Check sheet for the modelled part. Datum: model origin and axes. Units: mm. Round coordinates to 2 decimals unless told otherwise and drop trailing zeros. Answer in a Markdown table with one row per item. Add a question column.
(1) Gauge pin test, flat ends, axial feed: pin 1 (3.5 mm diameter, centred on x = 67.66, z = 82.18, fed in from -Y); pin 2 (3.5 mm diameter, centred on x = 83.14, z = -39.84, fed in from -Y); pin 3 (1.5 mm diameter, centred on x = 147.5, y = 2, fed in from +Z); pin 4 (0.9 mm diameter, centred on x = -133, y = 2, fed in from -Z). Record the tip position at first contact, or that the pin passes through.
(2) Cross-section at A-A on y = 1.85. Count the separate pieces of the cut face and the enclosed holes in it, then the cut area to 3 significant figures.
(3) Thickness scan on line 1 along Z through (x, y) = (70, 1.55); line 2 along Z through (x, y) = (-50, 1.8); line 3 along X through (y, z) = (0.6, 118). Record the ranges inside material, lowest first.
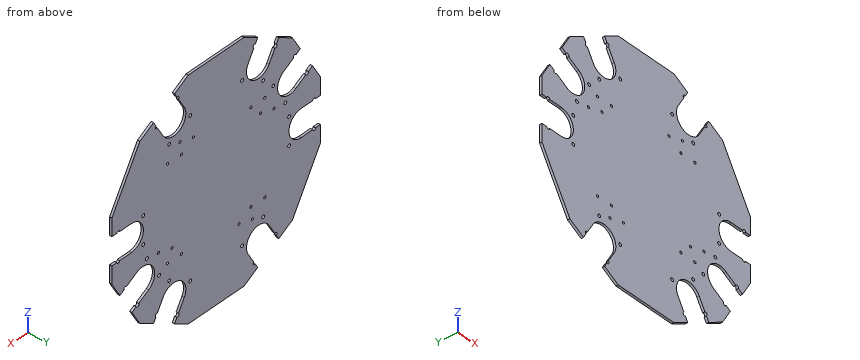
from build123d import *

# Parameters (mm, degrees)
BOSS_EXTRUDE1_DEPTH     = 3
SKETCH2_R               = 2.05
HEXCUT1_DEPTH           = 3
SKETCH5_R               = 1.55
RAILMOUNTHOLES_DEPTH    = 3
LPATTERN1_COUNT         = 2
LPATTERN1_PITCH         = 120
LPATTERN1_COUNT_DIR2    = 2
LPATTERN1_PITCH_DIR2    = 120
SKETCH6_R               = 2.05
QUADCUT1_DEPTH          = 3
CUT_EXTRUDE3_DEPTH      = 3
CUT_EXTRUDE4_DEPTH      = 3
SKETCH9_R               = 1.55
CUT_EXTRUDE5_DEPTH      = 3
MIRROR6_COPY_1_SKETCH_R = 1.55
MIRROR6_COPY_1_DEPTH    = 3
MIRROR6_COPY_2_SKETCH_R = 1.55
MIRROR6_COPY_2_DEPTH    = 3


with BuildPart() as part:
    # Sketch1 → Boss-Extrude1 (new body)
    with BuildSketch(Plane(origin=(0, 0, 0), x_dir=(1, 0, 0), z_dir=(0, 1, 0))):
        Polygon((150, -40.192378865), (150, 40.192378865), (109.807621135, 109.807621135), (40.192378865, 150), (-40.192378865, 150), (-109.807621135, 109.807621135), (-150, 40.192378865), (-150, -40.192378865), (-109.807621135, -109.807621135), (-40.192378865, -150), (40.192378865, -150), (109.807621135, -109.807621135), align=None)
    extrude(amount=BOSS_EXTRUDE1_DEPTH)

    # Sketch2 → HexCut1 (cut)
    with BuildSketch(Plane(origin=(0, 3, 0), x_dir=(1, 0, 0), z_dir=(0, 1, 0))):
        with Locations(Location((55.344555434, 130.859581934, 0), (0, 0, 270))):
            Circle(SKETCH2_R)
        with Locations(Location((37.344555434, 99.682667397, 0), (0, 0, 270))):
            Circle(SKETCH2_R)
        with Locations(Location((37.344555434, -99.682667397, 0), (0, 0, 270))):
            Circle(SKETCH2_R)
        with Locations(Location((55.344555434, -130.859581934, 0), (0, 0, 270))):
            Circle(SKETCH2_R)
        with Locations(Location((105, 17.5, 0), (0, 0, 270))):
            Circle(SKETCH2_R)
        with Locations(Location((141, 17.5, 0), (0, 0, 270))):
            Circle(SKETCH2_R)
        with Locations(Location((105, -17.5, 0), (0, 0, 270))):
            Circle(SKETCH2_R)
        with Locations(Location((141, -17.5, 0), (0, 0, 270))):
            Circle(SKETCH2_R)
        with Locations(Location((85.655444566, -113.359581934, 0), (0, 0, 270))):
            Circle(SKETCH2_R)
        with Locations(Location((67.655444566, -82.182667397, 0), (0, 0, 270))):
            Circle(SKETCH2_R)
        with Locations(Location((85.655444566, 113.359581934, 0), (0, 0, 270))):
            Circle(SKETCH2_R)
        with Locations(Location((67.655444566, 82.182667397, 0), (0, 0, 270))):
            Circle(SKETCH2_R)
    hexcut1 = extrude(amount=-HEXCUT1_DEPTH, mode=Mode.SUBTRACT)

    # HexCut2: HexCut1 across plane
    add(hexcut1.mirror(Plane(origin=(0, 0, 0), x_dir=(0, 0, 1), z_dir=(1, 0, 0))), mode=Mode.SUBTRACT)

    # Sketch5 → RailMountHoles (cut)
    with BuildSketch(Plane(origin=(0, 3, 0), x_dir=(1, 0, 0), z_dir=(0, 1, 0))):
        with Locations(Location((50, 60, 0), (0, 0, 270))):
            Circle(SKETCH5_R)
        with Locations(Location((70, 60, 0), (0, 0, 270))):
            Circle(SKETCH5_R)
    railmountholes = extrude(amount=-RAILMOUNTHOLES_DEPTH, mode=Mode.SUBTRACT)

    # LPattern1: RailMountHoles 2 × 2
    with Locations(*[(-j * LPATTERN1_PITCH_DIR2, 0, i * LPATTERN1_PITCH) for i in range(LPATTERN1_COUNT) for j in range(LPATTERN1_COUNT_DIR2) if (i, j) != (0, 0)]):
        add(railmountholes, mode=Mode.SUBTRACT)

    # Sketch6 → QuadCut1 (cut)
    with BuildSketch(Plane(origin=(0, 3, 0), x_dir=(1, 0, 0), z_dir=(0, 1, 0))):
        with Locations(Location((99.682667397, 37.344555434, 0), (0, 0, 270))):
            Circle(SKETCH6_R)
        with Locations(Location((130.859581934, 55.344555434, 0), (0, 0, 270))):
            Circle(SKETCH6_R)
        with Locations(Location((113.359581934, 85.655444566, 0), (0, 0, 270))):
            Circle(SKETCH6_R)
        with Locations(Location((82.182667397, 67.655444566, 0), (0, 0, 270))):
            Circle(SKETCH6_R)
    quadcut1 = extrude(amount=-QUADCUT1_DEPTH, mode=Mode.SUBTRACT)

    # Mirror1: QuadCut1 across plane
    add(quadcut1.mirror(Plane(origin=(0, 0, 0), x_dir=(0.5000000000000011, 0, 0.8660254037844378), z_dir=(0.8660254037844379, 0, -0.5000000000000012))), mode=Mode.SUBTRACT)

    # Sketch7 → Cut-Extrude3 (cut)
    with BuildSketch(Plane(origin=(0, 3, 0), x_dir=(1, 0, 0), z_dir=(0, 1, 0))):
        with BuildLine():
            Line((45.994555434, 114.664906883), (83.494555434, 179.616812167))
            Line((83.494555434, 179.616812167), (113.805444566, 162.116812167))
            Line((113.805444566, 162.116812167), (76.305444566, 97.164906883))
            ThreePointArc((76.305444566, 97.164906883), (52.4, 90.759462317), (45.994555434, 114.664906883))
        make_face()
        with BuildLine():
            Line((45.994555434, -114.664906883), (83.494555434, -179.616812167))
            Line((83.494555434, -179.616812167), (113.805444566, -162.116812167))
            Line((113.805444566, -162.116812167), (76.305444566, -97.164906883))
            ThreePointArc((76.305444566, -97.164906883), (52.4, -90.759462317), (45.994555434, -114.664906883))
        make_face()
        with BuildLine():
            Line((122.3, 17.5), (162.3, 17.5))
            Line((162.3, 17.5), (162.3, -17.5))
            Line((162.3, -17.5), (122.3, -17.5))
            ThreePointArc((122.3, -17.5), (104.8, 0), (122.3, 17.5))
        make_face()
    cut_extrude3 = extrude(amount=-CUT_EXTRUDE3_DEPTH, mode=Mode.SUBTRACT)

    # Mirror2: Cut-Extrude3 across plane
    add(cut_extrude3.mirror(Plane(origin=(0, 0, 0), x_dir=(0, 0, 1), z_dir=(1, 0, 0))), mode=Mode.SUBTRACT)

    # Sketch8 → Cut-Extrude4 (cut)
    with BuildSketch(Plane(origin=(0, 3, 0), x_dir=(1, 0, 0), z_dir=(0, 1, 0))):
        with BuildLine():
            Line((97.164906883, 76.305444566), (131.805923034, 96.305444566))
            Line((131.805923034, 96.305444566), (149.305923034, 65.994555434))
            Line((149.305923034, 65.994555434), (114.664906883, 45.994555434))
            ThreePointArc((114.664906883, 45.994555434), (90.759462317, 52.4), (97.164906883, 76.305444566))
        make_face()
    cut_extrude4 = extrude(amount=-CUT_EXTRUDE4_DEPTH, mode=Mode.SUBTRACT)

    # Mirror3: Cut-Extrude4 across plane
    add(cut_extrude4.mirror(Plane(origin=(0, 0, 0), x_dir=(0.5000000000000011, 0, 0.8660254037844378), z_dir=(0.8660254037844379, 0, -0.5000000000000012))), mode=Mode.SUBTRACT)

    # Sketch9 → Cut-Extrude5 (cut)
    with BuildSketch(Plane(origin=(0, 3, 0), x_dir=(1, 0, 0), z_dir=(0, 1, 0))):
        with Locations(Location((63.825434021, 45.014597322, 0), (0, 0, 270))):
            Circle(SKETCH9_R)
        with Locations(Location((83.143950546, 39.83821642, 0), (0, 0, 270))):
            Circle(SKETCH9_R)
    cut_extrude5 = extrude(amount=-CUT_EXTRUDE5_DEPTH, mode=Mode.SUBTRACT)

    # Mirror4: Cut-Extrude5 across plane
    add(cut_extrude5.mirror(Plane(origin=(0, 0, 0), x_dir=(0.9659258262890692, 0, 0.2588190451025174), z_dir=(0.2588190451025174, 0, -0.9659258262890692))), mode=Mode.SUBTRACT)

    # Mirror5: Cut-Extrude5 across plane
    add(cut_extrude5.mirror(Plane(origin=(0, 0, 0), x_dir=(-0.2588190451025206, 0, 0.9659258262890683), z_dir=(0.9659258262890683, 0, 0.2588190451025206))), mode=Mode.SUBTRACT)

    # Mirror6 copy 1 sketch → Mirror6 copy 1 (cut)
    with BuildSketch(Plane(origin=(0, 3, 0), x_dir=(-1, 0, 0), z_dir=(0, 1, 0))):
        with Locations(Location((63.825434021, 45.014597322, 0), (0, 0, 270))):
            Circle(MIRROR6_COPY_1_SKETCH_R)
        with Locations(Location((83.143950546, 39.83821642, 0), (0, 0, 270))):
            Circle(MIRROR6_COPY_1_SKETCH_R)
    extrude(amount=-MIRROR6_COPY_1_DEPTH, mode=Mode.SUBTRACT)

    # Mirror6 copy 2 sketch → Mirror6 copy 2 (cut)
    with BuildSketch(Plane(origin=(0, 3, 0), x_dir=(-0.8660254037844388, 0, -0.49999999999999967), z_dir=(0, 1, 0))):
        with Locations((63.825434021, -45.014597322)):
            Circle(MIRROR6_COPY_2_SKETCH_R)
        with Locations((83.143950546, -39.83821642)):
            Circle(MIRROR6_COPY_2_SKETCH_R)
    extrude(amount=-MIRROR6_COPY_2_DEPTH, mode=Mode.SUBTRACT)


solid = part.part
Answers:
| question | item | result |
|---|---|---|
| 1 | pin 1 | passes through |
| 1 | pin 2 | stops at y = 0 |
| 1 | pin 3 | stops at z = 45.82 |
| 1 | pin 4 | stops at z = -70.42 |
| 2 | separate pieces | 1 |
| 2 | enclosed holes | 32 |
| 2 | area | 60,300 mm^2 |
| 3 | line 1 | z = -90.82 to -61.55, -58.45 to 58.45, 61.55 to 90.82 |
| 3 | line 2 | z = -144.34 to -121.6, -92.43 to -61.55, -58.45 to 58.45, 61.55 to 92.43, 121.6 to 144.34 |
| 3 | line 3 | x = -95.62 to -88.33, -47.92 to 47.92, 88.33 to 95.62 |
